CAD build for the part. Positions are in the model's coordinates, mm. A direction names the side the tool comes from. Round coordinates to 2 decimals unless told otherwise and drop trailing zeros. Order: outer loops, then holes, each group sorted by start corner. A loop starts at its lowest first (then second) coordinate and runs counter-clockwise, first axis right, second up. Notation, with made-up numbers: M 34,81 L 70,81 A15 cw 70,93 Z; hole C -16.75,79 d11. An arc over 180 degrees is marked long. Answer as a JSON object with one key per item and string values.
Solid Edge part; units mm, degrees
sketch "Sketch1" plane through (0, 0, 0) normal (0, 0, 1) x (1, 0, 0)
  line L0 (-23, 6.25) -> (-23, 7.5)
  line L1 (-23, 7.5) -> (-21, 7.5)
  line L2 (-21, 7.5) -> (-21, 5)
  line L3 (-29.0004, 5) -> (-21, 5)
  line L4 (-29.0004, 12) -> (-29.0004, 5)
  line L5 (-29.0004, 12) -> (-21, 12)
  line L6 (-21, 12) -> (-21, 9.5)
  line L7 (-21, 9.5) -> (-23, 9.5)
  line L8 (-23, 9.5) -> (-23, 10.75)
  line L9 (-23, 10.75) -> (-25, 10.75)
  line L10 (-25, 10.75) -> (-25, 6.25)
  line L11 (-25, 6.25) -> (-23, 6.25)
  line L12 (0, 17) -> (-50, 17)
  line L13 (-50, 17) -> (-50, 0)
  line L14 (-50, 0) -> (0, 0)
  line L15 (0, 0) -> (0, 17)
extrude "ProtrusiónExtruida_1" add sketch "Sketch1" along normal blind 40
sketch "Sketch2" plane through (-25, 0, 20) normal (0, -1, 0) x (1, 0, 0)
  line L0 (-5, -15) -> (5, -15)
  line L1 (5, -15) -> (5, 15)
  line L2 (5, 15) -> (-5, 15)
  line L3 (-5, 15) -> (-5, -15)
extrude "VaciadoExtruido_2" cut sketch "Sketch2" against normal blind 92
hole "Agujero_2" at (0, 8.5, 20) direction (-1, 0, 0) diameter 11.5 end up to next
fillet "Redondeo_1" radius 10 2 edges at (-50, 8.5, 0) (-50, 8.5, 40)
Item 1: Saw through at C-C on z = 26.5. List the corners of the cut face in (x, y).
Worked answers:
{"outline": "M -50,0 L -30,0 L -30,17 L -50,17 Z; M -20,0 L 0,0 L 0,17 L -20,17 Z"}
Item 2: 3-axis set-ups, long thin cutter, end or side, ignore diameter. For faces 5 (the flat face through (-19, 17, 20)), 6 (the flat face through (-29, 9, 2)), 7 (the flat face through (-20, 3, 23)): which of +Z, -Z, +X, -X, +Y, -Y reach the whole face in a straight line?
Worked answers:
{"face 5": "+Z, -Z, +X, -X, +Y", "face 6": "+Z, -Z", "face 7": "+Y, -Y"}
Item 3: Two-plate mould, pull along X, no slides. Class faces 1 (the flat face through (0, 5, 15)), 2 (the cylindrical face through (-47.15, 8.38, 3.01)), 3 (the flat face through (-23, 10, 37)), 4 (the flat face through (-20, 9, 0)): released by +X, released by -X, zero draft, split by the parting line, or undercut.
Worked answers:
{"face 1": "released by +X", "face 2": "released by -X", "face 3": "undercut", "face 4": "zero draft"}
Item 4: Drop flat-ended pins along their axis: pin 1 Ø0.8 at (y, z) = (10, 3.5) entering from -X; pin 2 Ø1.5 at (x, z) = (-22.5, 6.5) entering from -Y; pin 3 Ø0.8 at (y, z) = (10.5, 37.5) entering from -X. Give the stop position or say it passes through.
Worked answers:
{"pin 1": "stops at x = -47.92", "pin 2": "passes through", "pin 3": "stops at x = -47.04"}
Item 5: Saw through at A-A on z = 20. List the corners of the cut face in (x, y).
Worked answers:
{"outline": "M -50,0 L -30,0 L -30,17 L -50,17 Z; M -20,0 L 0,0 L 0,2.75 L -20,2.75 Z; M -20,14.25 L 0,14.25 L 0,17 L -20,17 Z"}
Item 6: Saw through at B-B on y = 8.5. List the corners of the cut face in (x, z), and give its area (3 significant figures).
Worked answers:
{"outline": "M -50,10 A10 ccw -40,0 L -29,0 L -29,5 L -30,5 L -30,35 L -29,35 L -29,40 L -40,40 A10 ccw -50,30 Z; M -25,0 L 0,0 L 0,14.25 L -20,14.25 L -20,5 L -25,5 Z; M -25,35 L -20,35 L -20,25.75 L 0,25.75 L 0,40 L -25,40 Z", "area": "1,390 mm2"}
Item 7: Wall check: line 1 along Y through (x, z) = (-21.5, 36); line 2 along X through (y, z) = (10.25, 9.5); line 3 along Y through (x, z) = (-5, 20). Give the ranges that are in metal, low to high. Write a range as [from, to].
Worked answers:
{"line 1": "y = [0, 5], [7.5, 9.5], [12, 17]", "line 2": "x = [-49.99, -30], [-20, 0]", "line 3": "y = [0, 2.75], [14.25, 17]"}
Item 8: Saw through at D-D on z = 36. List the corners of the cut face in (x, y).
Worked answers:
{"outline": "M -48,0 L 0,0 L 0,17 L -48,17 Z; hole M -29,5 L -21,5 L -21,7.5 L -23,7.5 L -23,6.25 L -25,6.25 L -25,10.75 L -23,10.75 L -23,9.5 L -21,9.5 L -21,12 L -29,12 Z"}
